Work out the finished part from the listing and answer in its coordinate system (mm). A direction names the side the tool comes from. Coordinates: 2 decimals unless noted, no trailing zeros. Order: outer loops, then holes, each group sorted by start corner. A loop starts at its lowest first (then second) coordinate and runs counter-clockwise, first axis right, second up. Notation, with made-up numbers: M -24.5,85 L -15.5,85 A16 cw -15.5,112 Z; hole C 0.25,47 d5. An arc over 180 degrees is marked long. Use a Markdown table: item, result.
from build123d import *

# Parameters (mm, degrees)
F0_W     = 36.83
F0_H     = 76.2
F1_DEPTH = 3.81
F2_W     = 8.89
F2_H     = 3.81
F3_DEPTH = 3.81
F4_W     = 8.89
F4_H     = 3.81
F5_DEPTH = 3.81
F6_R     = 4.9784
F7_DEPTH = 3.81


with BuildPart() as f1:
    # F0 (on Front) → F1 (new body)
    with BuildSketch(Plane.XZ):
        Polygon((-88.9, -66.0091239631), (0, -66.0091239631), (88.9, -66.0091239631), (88.9, 22.8908760369), (0, 92.7408760369), (-88.9, 22.8908760369), align=None)
        with Locations((-60.325, -15.2091239631)):
            Rectangle(F0_W, F0_H, mode=Mode.SUBTRACT)
        with Locations((60.325, -15.2091239631)):
            Rectangle(F0_W, F0_H, mode=Mode.SUBTRACT)
    extrude(amount=F1_DEPTH)

    # F2 (on face) → F3 (cut)
    with BuildSketch(Plane(origin=(-45.0539271599, 0, 57.3413618398), x_dir=(0.7863183388, 0, 0.6178215519), z_dir=(-0.6178215519, 0, 0.7863183388))):
        with Locations((-14.4576880394, -1.905)):
            Rectangle(F2_W, F2_H)
        with Locations((23.6423119606, -1.905)):
            Rectangle(F2_W, F2_H)
        with Locations((42.6923119606, -1.905)):
            Rectangle(F2_W, F2_H)
        with Locations((4.5923119606, -1.905)):
            Rectangle(F2_W, F2_H)
    extrude(amount=-F3_DEPTH, mode=Mode.SUBTRACT)

    # F4 (on face) → F5 (cut)
    with BuildSketch(Plane(origin=(45.0539271599, 0, 57.3413618398), x_dir=(0.7863183388, 0, -0.6178215519), z_dir=(0.6178215519, 0, 0.7863183388))):
        with Locations((-42.6923119606, -1.905)):
            Rectangle(F4_W, F4_H)
        with Locations((-23.6423119606, -1.905)):
            Rectangle(F4_W, F4_H)
        with Locations((-4.5923119606, -1.905)):
            Rectangle(F4_W, F4_H)
        with Locations((14.4576880394, -1.905)):
            Rectangle(F4_W, F4_H)
    extrude(amount=-F5_DEPTH, mode=Mode.SUBTRACT)

    # F6 (on face) → F7 (cut)
    with BuildSketch(Plane(origin=(0, 0, 0), x_dir=(-1, 0, 0), z_dir=(0, 1, 0))):
        with Locations((0, 69.9647201129)):
            Circle(F6_R)
    extrude(amount=-F7_DEPTH, mode=Mode.SUBTRACT)


solid = f1.part
(1) Which of the six approach directions +Z, -Z, +X, -X, +Y, -Y give full straight-line access (tool end or side, diameter ignored) to faces 4 (the flat face through (-54.117, -1.878, 45.375)), 5 (the flat face through (88.9, -2, -22))?
Conclusion:
| item | result |
|---|---|
| face 4 | +Y, -Y |
| face 5 | +Z, -Z, +X, +Y, -Y |
(2) A cutting plane is placed at C-C (x = -71). Determine the outline of the cut face in (y, z).
Conclusion:
| item | result |
|---|---|
| outline | M -3.81,-66.01 L 0,-66.01 L 0,-53.31 L -3.81,-53.31 Z; M -3.81,22.89 L 0,22.89 L 0,36.96 L -3.81,36.96 Z |
(3) A cutting plane is placed at A-A (z = -8.5). Determine the outline of the cut face in (x, y).
Conclusion:
| item | result |
|---|---|
| outline | M -88.9,-3.81 L -78.74,-3.81 L -78.74,0 L -88.9,0 Z; M -41.91,-3.81 L 41.91,-3.81 L 41.91,0 L -41.91,0 Z; M 78.74,-3.81 L 88.9,-3.81 L 88.9,0 L 78.74,0 Z |
(4) A cutting plane is placed at B-B (x = 66.5). Determine the outline of the cut face in (y, z), then the cut area to 3 significant figures.
Conclusion:
| item | result |
|---|---|
| outline | M -3.81,-66.01 L 0,-66.01 L 0,-53.31 L -3.81,-53.31 Z; M -3.81,22.89 L 0,22.89 L 0,40.49 L -3.81,40.49 Z |
| area | 115 mm2 |
(5) Determine the mould class of faces 1 (the flat face through (-33.897, -1.878, 66.107)), 2 (the flat face through (-78.74, -2, -16)), 3 (the flat face through (-1, -2, -66.009)) for opening direction Z: pulls with the +Z half, pulls with the -Z half, needs draft (parallel to the pull), parting line crosses it, or undercut.
Conclusion:
| item | result |
|---|---|
| face 1 | pulls with the +Z half |
| face 2 | undercut |
| face 3 | pulls with the -Z half |
(6) Straight lines are drawn through the part: L1, parallel to X at y = -0.4, z = 21; L2, parallel to Z at x = 0, y = -0.9; L3, parallel to X at y = -2.35, z = 44. For each, find the intervals that lie inside material, in ascending order.
Conclusion:
| item | result |
|---|---|
| L1 | -88.9 to -78.74, -41.91 to 41.91, 78.74 to 88.9 |
| L2 | -66.01 to 64.99, 74.94 to 92.74 |
| L3 | -62.03 to -58.61, -55.87 to 55.87, 58.61 to 62.03 |
(7) A cutting plane is placed at D-D (y = -2). Give the number of separate pieces and of enclosed holes in the cut face, then the cut area to 3 significant figures.
Conclusion:
| item | result |
|---|---|
| separate pieces | 1 |
| enclosed holes | 3 |
| area | 16,100 mm2 |
(8) Given P1, Ø1.9, axis at x = -58.5, y = -2, coming from the +Z side; P2, Ø1.1, axis at x = 55.5, y = -1, coming from the +Z side, each flat-ended and moving along its own axis, determine where each tip first touches the part or whether it passes through.
Conclusion:
| item | result |
|---|---|
| P1 | z = 45.07 |
| P2 | z = 44.72 |
